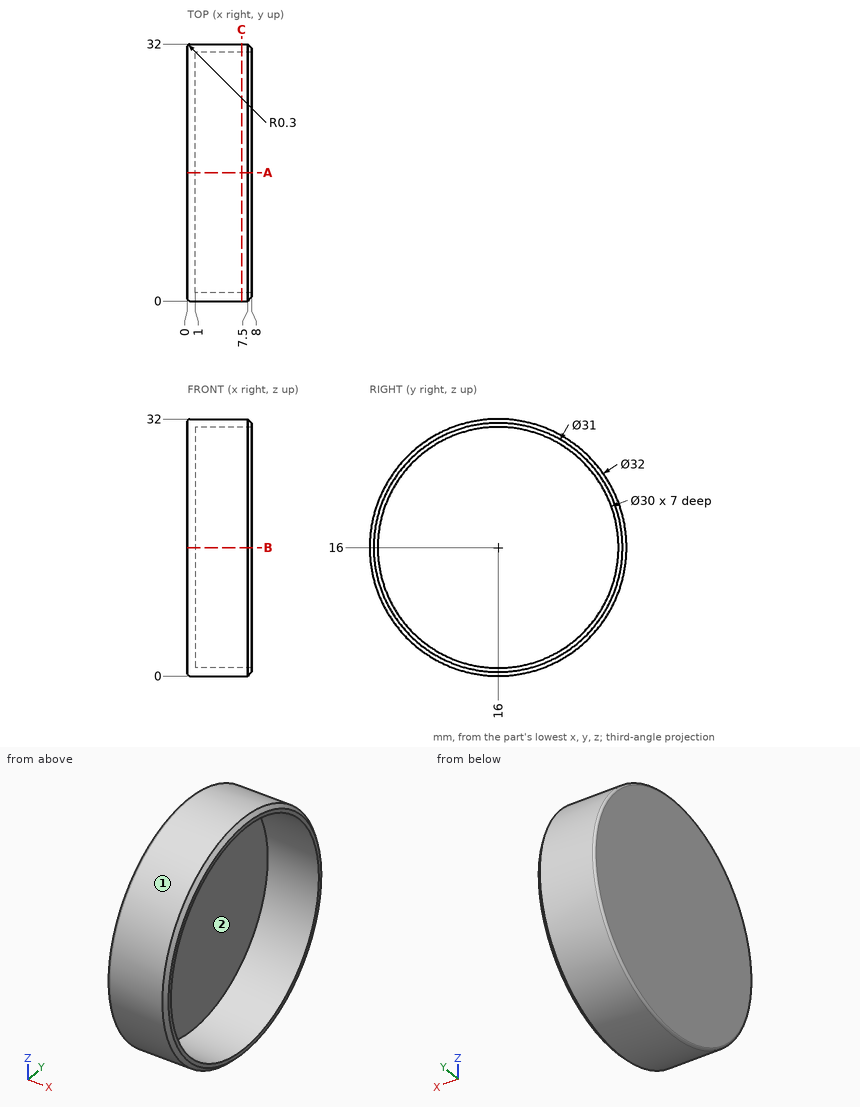
Could you check a few things on this drawing? It's one solid part, dimensions in mm from its lowest x, y, z. A direction names the side the tool comes from. Give positions to 0.01 mm unless a question says otherwise; leave off trailing zeros. Loops run counter-clockwise (first coordinate to the right, second up) from the corner with the lowest first, then second, coordinate; pieces in that order, holes last. Notation, with made-up numbers: (51.5, 12) -> (107.5, 12) arc R13 cw to (107.5, 33) -> close; hole circle Ø11 at (-6, 56). An arc over 180 degrees is marked (long way). Use one line per item in the form item = value. Start each with the question number.
1) Imagine slicing it at C-C (x = 6.75). Please give me the cut outline in (y, z), then the cut area to 3 significant figures.
2) Which directions (+Z, -Z, +X, -X, +Y, -Y) give clear straight access to the entire face, cutting with the end or side of a thin tool? Please do the marked faces 1 and 2.
3) Please list where these lines run through material, in increasing order: line 1 along Y through (x, z) = (6, 16); line 2 along X through (y, z) = (25, 13).
4) For P1, Ø18, axis at y = 16, z = 16, coming from the +X side; P2, Ø3, axis at x = 3, y = 20, coming from the -Z side, each with a flat end and sliding along its axis, tell me the tip position at first contact or that it passes through.
5) Imagine slicing it at A-A (y = 16). Please give me the cut outline in (x, z).
Check values:
q1.outline = circle Ø32 at (16, 16); hole circle Ø30 at (16, 16)
q1.area = 97.4 mm^2
q2.face_1 = +X, -X
q2.face_2 = +X
q3.line_1 = 0 to 1, 31 to 32
q3.line_2 = 0 to 1
q4.P1 = 1
q4.P2 = 0.2
q5.outline = (0, 0.3) arc R0.3 ccw to (0.3, 0) -> (7.5, 0) -> (8, 0.5) -> (8, 1) -> (1, 1) -> (1, 31) -> (8, 31) -> (8, 31.5) -> (7.5, 32) -> (0.3, 32) arc R0.3 ccw to (0, 31.7) -> close
